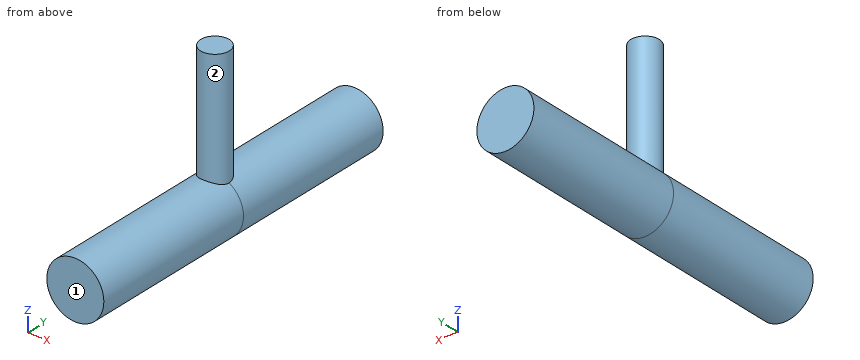
from build123d import *

# Parameters (mm, degrees)
F1_R     = 3.175
F2_DEPTH = 31.75
F0_R     = 6.35
F3_DEPTH = 38.1
F4_DEPTH = 38.1


with BuildPart() as f2:
    # F1 (on Top) → F2 (new body)
    with BuildSketch(Plane.XY):
        Circle(F1_R)
    extrude(amount=F2_DEPTH)

    # F0 (on Front) → F3 (join)
    with BuildSketch(Plane.XZ):
        Circle(F0_R)
    extrude(amount=F3_DEPTH)

    # F0 (on Front) → F4 (join)
    with BuildSketch(Plane.XZ):
        Circle(F0_R)
    extrude(amount=-F4_DEPTH)


solid = f2.part
Can you work these out from the model? Positions are in its coordinate system, mm. Face numbers are marked on the shaded views. A direction names the side the tool comes from. Round coordinates to 2 decimals unless told otherwise and drop trailing zeros. Order: outer loops, then holes, each group sorted by start corner. A loop starts at its lowest first (then second) coordinate and runs counter-clockwise, first axis right, second up. Notation, with made-up numbers: (-5.5, -25.75) -> (39.5, -25.75) arc R17 cw to (39.5, -3.75) -> close; hole circle Ø5 at (-12.5, -39.5). An arc over 180 degrees is marked (long way). Write each question's results on one line, items separated by ' | '. Start each with the question number.
Item 1: If we section it at B-B, the plane y = -26.5: Write out the boundary of the cut face in (x, z), then the cut area to 3 significant figures.
Item 2: Will these pins go through, and if not, where does the flat tip stop? pin 1 (2 mm diameter, centred on x = -2.5, z = 25, fed in from -Y); pin 2 (4 mm diameter, centred on x = 3.5, z = 20.5, fed in from +Y); pin 3 (3 mm diameter, centred on x = -5, y = 13, fed in from +Z).
Item 3: If we section it at C-C, the plane z = 18: Write out the boundary of the cut face in (x, y) (3 decimals).
Item 4: If we section it at A-A, the plane x = 0: Write out the boundary of the cut face in (y, z) (3 decimals).
Item 5: Which directions (+Z, -Z, +X, -X, +Y, -Y) give clear straight access to the entire face, cutting with the end or side of a thin tool? Please do the marked faces 1 and 2.
Item 6: If we section it at D-D, the plane x = 5: Write out the boundary of the cut face in (y, z), then the cut area to 3 significant figures.
Item 7: Please list where these lines run through material, in increasing order: L1, parallel to Z at x = 0, y = 9.5; L2, parallel to Y at x = -2.75, z = 11.5; L3, parallel to X at y = -10.5, z = -3.
Results:
1) outline: circle Ø12.7 at (0, 0) | area: 127 mm2
2) pin 1: stops at y = -2.8 | pin 2: stops at y = 2.8 | pin 3: stops at z = 5.3
3) outline: circle Ø6.35 at (0, 0)
4) outline: (-38.1, -6.35) -> (38.1, -6.35) -> (38.1, 6.35) -> (3.175, 6.35) -> (3.175, 31.75) -> (-3.175, 31.75) -> (-3.175, 6.35) -> (-38.1, 6.35) -> close
5) face 1: +Z, -Z, +X, -X, -Y | face 2: +Z
6) outline: (-38.1, -3.91) -> (38.1, -3.91) -> (38.1, 3.91) -> (-38.1, 3.91) -> close | area: 597 mm2
7) L1: z = -6.35 to 6.35 | L2: y = -1.59 to 1.59 | L3: x = -5.6 to 5.6
